from build123d import *

# Parameters (mm, degrees)
BOSS_EXTRUDE1_DEPTH = 2
SKETCH2_W           = 20
SKETCH2_H           = 6.2
BOSS_EXTRUDE2_DEPTH = 36
BOSS_EXTRUDE3_DEPTH = 5


with BuildPart() as part:
    # Sketch1 → Boss-Extrude1 (new body)
    with BuildSketch(Plane(origin=(0, 0, 0), x_dir=(0, 0, -1), z_dir=(1, 0, 0))):
        Polygon((-43, 47.5), (43, 47.5), (43, 32.5), (0, -47.5), (-43, 32.5), align=None)
    extrude(amount=BOSS_EXTRUDE1_DEPTH)

    # Sketch2 → Boss-Extrude2 (add)
    with BuildSketch(Plane(origin=(2, 0, 0), x_dir=(0, 0, -1), z_dir=(1, 0, 0))):
        with Locations((0, 34.4)):
            Rectangle(SKETCH2_W, SKETCH2_H)
    extrude(amount=BOSS_EXTRUDE2_DEPTH)

    # Sketch3 → Boss-Extrude3 (add, symmetric)
    with BuildSketch(Plane.XY):
        Polygon((2, 19.36818927), (25.86362146, 31.3), (12, 31.3), (2, 26.3), align=None)
    extrude(amount=BOSS_EXTRUDE3_DEPTH, both=True)


solid = part.part
Model file for the job. Use its own axes, mm. A direction names the side the tool comes from. Coordinates: 2 decimals unless noted, no trailing zeros. Order: outer loops, then holes, each group sorted by start corner. A loop starts at its lowest first (then second) coordinate and runs counter-clockwise, first axis right, second up. Notation, with made-up numbers: M 55,35.5 L 77,35.5 A25 ccw 77,57.5 Z; hole C 37,79 d11. An arc over 180 degrees is marked long. Return JSON: item names as keys, results as strings.
1. Flat gauge pins, fed straight in: pin 1 (13 mm diameter, centred on x = 16.5, y = 25.5, fed in from -Z); pin 2 (3 mm diameter, centred on x = 20.5, y = 28.5, fed in from +Z); pin 3 (1.9 mm diameter, centred on x = 22, y = 35, fed in from +Z). Where does each tip first touch, or does it go through?
Ans:
{"pin 1": "z = -10", "pin 2": "z = 5", "pin 3": "z = 10"}
2. Tool access for faces 4 (the face through (11, 27, -5)), 5 (the face through (20, 37.5, 0)), 6 (the face through (20, 34, 10)): list every direction of +Z, -Z, +X, -X, +Y, -Y with a clear straight run to the whole face (end or side of a thin tool).
Ans:
{"face 4": "-Z, +X, -Y", "face 5": "+Z, -Z, +X, +Y", "face 6": "+Z, +X, +Y, -Y"}
3. Drill centre lines: probe 1 along X at (y, z) = (8, 5.5); probe 2 along Z at (x, y) = (25.5, 33); probe 3 along Y at (x, z) = (11, -9). Where is each one in solid material? Low to high.
Ans:
{"probe 1": "0 to 2", "probe 2": "-10 to 10", "probe 3": "31.3 to 37.5"}
4. Saw through at C-C (x = 21). Give the cut face in (y, z).
Ans:
{"outline": "M 28.87,-5 L 31.3,-5 L 31.3,-10 L 37.5,-10 L 37.5,10 L 31.3,10 L 31.3,5 L 28.87,5 Z"}
5. Pull direction X, two halves, no side cores. Call faces 1 (the face through (20, 31.3, 7)), 2 (the face through (0, 11, -1)), 3 (the face through (20, 34, -10)): +X half, -X half, draft (parallel to the pull), parting line (faces both ways), or undercut.
Ans:
{"face 1": "undercut", "face 2": "-X half", "face 3": "draft"}
6. Saw through at D-D (z = -37). Give the cut face in (x, y), and give its area (3 significant figures).
Ans:
{"outline": "M 0,21.34 L 2,21.34 L 2,47.5 L 0,47.5 Z", "area": "52.3 mm^2"}
7. Saw through at A-A (x = 9). Give the cut face in (y, z).
Ans:
{"outline": "M 22.87,-5 L 29.8,-5 L 29.8,5 L 22.87,5 Z; M 31.3,-10 L 37.5,-10 L 37.5,10 L 31.3,10 Z"}
8. Saw through at B-B (y = 41). Give the cut face in (x, z), and give its area (3 significant figures).
Ans:
{"outline": "M 0,-43 L 2,-43 L 2,43 L 0,43 Z", "area": "172 mm^2"}
